from build123d import *

# Parameters (mm, degrees)
IZIM1_R                     = 210
IZIM1_R_2                   = 12.55
IZIM1_W                     = 73
IZIM1_H                     = 73
Y_KSEKLIK_EKSTR_ZYON1_DEPTH = 10


with BuildPart() as part:
    # Çizim1 → Yükseklik-Ekstrüzyon1 (new body)
    with BuildSketch(Plane.XY):
        Circle(IZIM1_R)
        with Locations((0, 165)):
            Circle(IZIM1_R_2, mode=Mode.SUBTRACT)
        with Locations((165, 0)):
            Circle(IZIM1_R_2, mode=Mode.SUBTRACT)
        with Locations((0, -165)):
            Circle(IZIM1_R_2, mode=Mode.SUBTRACT)
        with Locations((-165, 0)):
            Circle(IZIM1_R_2, mode=Mode.SUBTRACT)
        Rectangle(IZIM1_W, IZIM1_H, mode=Mode.SUBTRACT)
    extrude(amount=Y_KSEKLIK_EKSTR_ZYON1_DEPTH)


solid = part.part
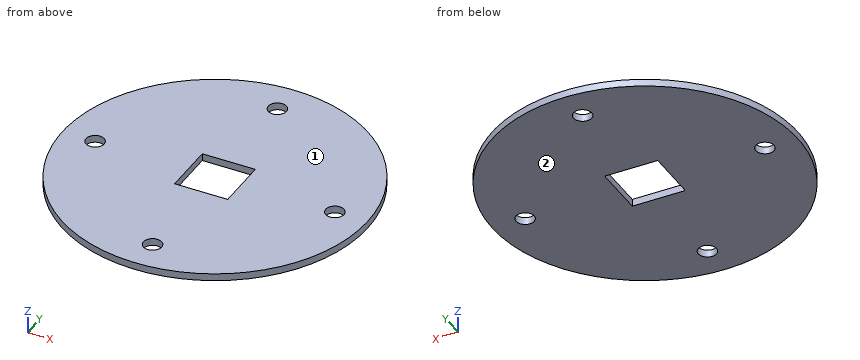
The model under review builds one solid part; all positions refer to its coordinate system, in mm. Face numbers are marked on the shaded views. Coordinates: 2 decimals unless noted, no trailing zeros. Order: outer loops, then holes, each group sorted by start corner. A loop starts at its lowest first (then second) coordinate and runs counter-clockwise, first axis right, second up. Notation, with made-up numbers: (54.25, 77) -> (83.25, 77) arc R27 ccw to (83.25, 101) -> close; hole circle Ø8 at (4, 8). An arc over 180 degrees is marked (long way). Answer in a Markdown table with one row per item.
(1) Consider section A-A (y = 0). Write out the cut boundary in (x, z).
Answers:
| item | result |
|---|---|
| outline | (-210, 0) -> (-177.55, 0) -> (-177.55, 10) -> (-210, 10) -> close; (-152.45, 0) -> (-36.5, 0) -> (-36.5, 10) -> (-152.45, 10) -> close; (36.5, 0) -> (152.45, 0) -> (152.45, 10) -> (36.5, 10) -> close; (177.55, 0) -> (210, 0) -> (210, 10) -> (177.55, 10) -> close |
(2) Insertion check: pin 1 (22.5 mm diameter, centred on x = 165, y = 0, fed in from +Z); pin 2 (3 mm diameter, centred on x = -31, z = 8, fed in from +Y); pin 3 (4 mm diameter, centred on x = 23, z = 1.5, fed in from -Y); pin 4 (5 mm diameter, centred on x = 105.5, z = 6, fed in from -Y). Each pin has a flat end and moves straight along its axis. Give the tip position at first contact, or say it passes through.
Answers:
| item | result |
|---|---|
| pin 1 | through |
| pin 2 | y = 207.92 |
| pin 3 | y = -208.95 |
| pin 4 | y = -183.01 |
(3) Consider section C-C (z = 6.75). Write out the cut boundary in (x, y), plus the area to 3 significant figures.
Answers:
| item | result |
|---|---|
| outline | circle Ø420 at (0, 0); hole circle Ø25.1 at (-165, 0); hole (-36.5, -36.5) -> (36.5, -36.5) -> (36.5, 36.5) -> (-36.5, 36.5) -> close; hole circle Ø25.1 at (0, -165); hole circle Ø25.1 at (0, 165); hole circle Ø25.1 at (165, 0) |
| area | 131,000 mm² |
(4) Wall thickness on line 1 along Y through (x, z) = (0, 5.25); line 2 along Y through (x, z) = (6, 7); line 3 along Y through (x, z) = (153.5, 1.5): over which ranges is each line inside the solid? List them lowest first.
Answers:
| item | result |
|---|---|
| line 1 | -210 to -177.55, -152.45 to -36.5, 36.5 to 152.45, 177.55 to 210 |
| line 2 | -209.91 to -176.02, -153.98 to -36.5, 36.5 to 153.98, 176.02 to 209.91 |
| line 3 | -143.31 to -5.03, 5.03 to 143.31 |
(5) The part is to be moulded in two halves that separate along Z. For the marked faces 1 and 2, say which applies: +Z half, -Z half, draft (parallel to the pull), parting line (faces both ways), or undercut.
Answers:
| item | result |
|---|---|
| face 1 | +Z half |
| face 2 | -Z half |
(6) Consider section D-D (y = -165). Write out the cut boundary in (x, z).
Answers:
| item | result |
|---|---|
| outline | (-129.9, 0) -> (-12.55, 0) -> (-12.55, 10) -> (-129.9, 10) -> close; (12.55, 0) -> (129.9, 0) -> (129.9, 10) -> (12.55, 10) -> close |
